Can you work these out from the drawing? Everything is in mm from the part's minimum corner. Round coordinates to 2 decimals unless told otherwise and drop trailing zeros. Loops run counter-clockwise (first coordinate to the right, second up) from the corner with the lowest first, then second, coordinate; pieces in that order, holes last. Notation, with made-up numbers: M 39.5,-34.5 L 61.5,-34.5 A17 cw 61.5,-5.5 Z; hole C -33.5,48.5 d10. An arc over 180 degrees is marked long. Use a Markdown table: item, result.
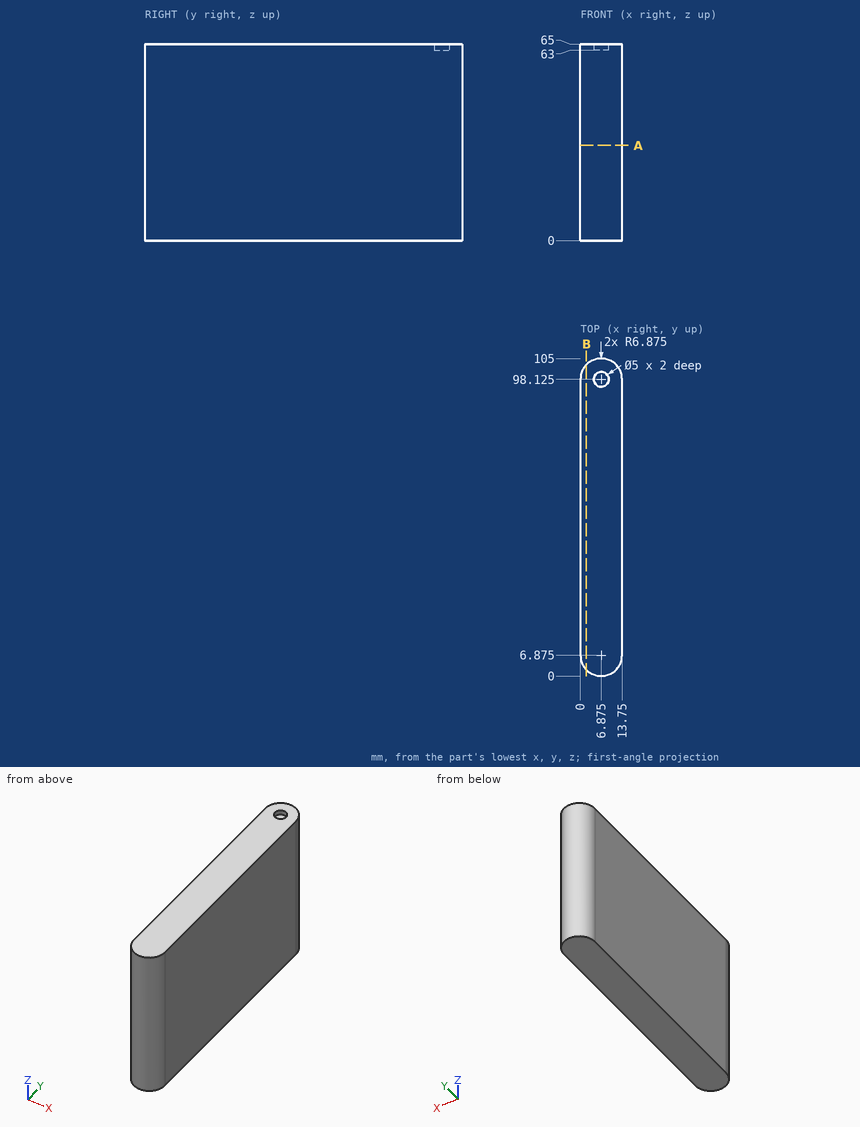
1. I need wall thicknesses on probe 1 along Y at (x, z) = (8.25, 29.5); probe 2 along Y at (x, z) = (12.75, 12); probe 3 along X at (y, z) = (6, 51.5). Which ranges of each line are inside material? Lowest first, please. Write a range as from..to.
Answer sheet:
| item | result |
|---|---|
| probe 1 | 0.14..104.86 |
| probe 2 | 3.3..101.7 |
| probe 3 | 0.06..13.69 |
2. Imagine slicing it at A-A, the plane z = 31.5. Write out the boundary of the cut face in (x, y) (3 decimals), then the cut area to 3 significant figures.
Answer sheet:
| item | result |
|---|---|
| outline | M 0,6.875 A6.875 ccw 13.75,6.875 L 13.75,98.125 A6.875 ccw 0,98.125 Z |
| area | 1,400 mm2 |
3. Imagine slicing it at B-B, the plane x = 2. Write out the boundary of the cut face in (y, z).
Answer sheet:
| item | result |
|---|---|
| outline | M 2.03,0 L 102.97,0 L 102.97,65 L 2.03,65 Z |
